Can you work these out from the model? Positions are in its coordinate system, mm. A direction names the side the tool comes from. Give positions to 0.01 mm unless a question says otherwise; leave off trailing zeros. Write each loop counter-clockwise with the first axis right and the second up, starting at its lowest first coordinate (ties: lowest second). Pieces come first, ordered by that corner, then holes.
Autodesk Inventor part; units mm, degrees
ref_plane "Work Plane2" through (0, 127, 0) normal (1, 0, 0) x (0, 0, -1)
ref_plane "YZ Plane" through (0, 0, 0) normal (1, 0, 0) x (0, 1, 0)
ref_plane "XZ Plane" through (0, 0, 0) normal (0, 1, 0) x (-1, 0, 0)
sketch "Sketch1" plane through (0, 0, 0) normal (0, 1, 0) x (-1, 0, 0)
  line L0 (16.4978, 9.525) -> (16.4978, -9.525)
  line L1 (16.4978, -9.525) -> (0, -19.05)
  line L2 (0, -19.05) -> (-16.4978, -9.525)
  line L3 (-16.4978, 9.525) -> (-16.4978, -9.525)
  line L4 (-16.4978, 9.525) -> (0, 19.05)
  line L5 (0, 19.05) -> (16.4978, 9.525)
  circle A0 centre (0, 0) radius 19.05 construction
  line L6 (0, 25.4) -> (0, -25.4) construction
  circle A1 centre (0, 0) radius 6.35
  dimension "d0" = 38.1
  dimension "d8" = 12.7
extrude "Hexagon1" add sketch "Sketch1" along normal blind 127 contours L0 L1 L2 L3 L4 L5 | A1
sketch "Sketch2" plane through (0, 127, 0) normal (0, 1, 0) x (1, 0, 0)
  circle A0 centre (0, 0) radius 6.35
  line L0 (0, 0) -> (25.4, 0) construction
  dimension "d3" = 12.7
ref_plane "Work Plane2" through (0, 127, 0) normal (1, 0, 0) x (0, 0, -1)
sketch "Sketch5" plane through (0, 127, 0) normal (1, 0, 0) x (0, 0, -1)
  line L0 (9.525, 0) -> (-9.525, 0)
  line L1 (0, 0) -> (0, 25.4)
  point P0 (0, -127)
  dimension "d9" = 25.4
sweep "Sweep1" add profiles "Sketch2" path "Sketch5" path curves L1
chamfer "Chamfer1" distance 3.175 angle 45 7 edges at (8.2489, 127, -14.2875) (-6.35, 127, 0) (16.4978, 127, 0) (8.2489, 127, 14.2875) (-8.2489, 127, -14.2875) (-16.4978, 127, 0) (-8.2489, 127, 14.2875)
properties part number "HexShaft1"
(1) Imagine slicing it at C-C, the plane x = 11.5. Write out the boundary of the cut face in (y, z) (3 decimals), plus the area to 3 significant figures.
Returned:
outline: (0, -12.41) - (123.825, -12.41) - (127, -8.744) - (127, 8.744) - (123.825, 12.41) - (0, 12.41) - close
area: 3,140 mm2
(2) Imagine slicing it at B-B, the plane y = 31. Write out the boundary of the cut face in (x, z) (3 decimals), plus the area to 3 significant figures.
Returned:
outline: (-16.498, -9.525) - (0, -19.05) - (16.498, -9.525) - (16.498, 9.525) - (0, 19.05) - (-16.498, 9.525) - close
area: 943 mm2
(3) Will these pins go through, and if not, where does the flat tip stop? P1, Ø1, axis at x = 2, y = 73.5, coming from the -Z side; P2, Ø3, axis at x = 10, y = 31, coming from the -Z side; P3, Ø3, axis at x = -4.5, y = 118.5, coming from the -Z side.
Returned:
P1: stops at z = -18.18
P2: stops at z = -14.14
P3: stops at z = -17.32
(4) Imagine slicing it at D-D, the plane y = 138.5. Write out the boundary of the cut face in (x, z).
Returned:
outline: circle Ø12.7 at (0, 0)
(5) For faces 1 (the face through (0, 127, -10)), 2 (the face through (-14.89, 125.43, -0.13)), which set-ups out of +Z, -Z, +X, -X, +Y, -Y let a thin tool reach every point of the face, with its end or its side?
Returned:
face 1: +Y
face 2: +Z, -Z, -X, +Y
(6) If I drill on L1, parallel to Y at x = -7.5, z = -7.5; L2, parallel to Z at x = 12, y = 26.5; L3, parallel to Z at x = -7, y = 64.5, over which ranges is the centre line in solid material (lowest first)?
Returned:
L1: y = 0 to 127
L2: z = -12.12 to 12.12
L3: z = -15.01 to 15.01
(7) Imagine slicing it at A-A, the plane z = 0. Write out the boundary of the cut face in (x, y) (3 decimals).
Returned:
outline: (-16.498, 0) - (16.498, 0) - (16.498, 123.825) - (13.323, 127) - (9.525, 127) - (6.35, 130.175) - (6.35, 152.4) - (-6.35, 152.4) - (-6.35, 130.175) - (-9.525, 127) - (-13.323, 127) - (-16.498, 123.825) - close
